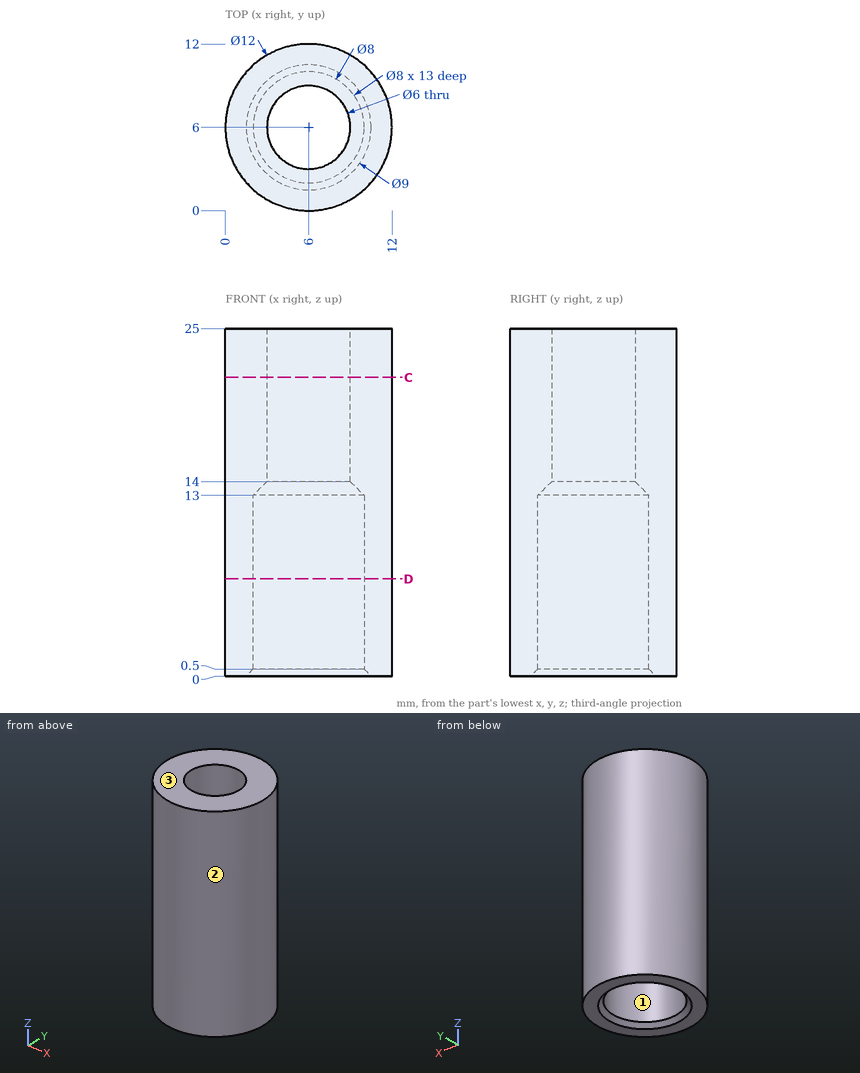
Here's the drawing with two shaded views (mm, measured from the low corner). I have some questions. Give positions to 0.01 mm unless a question says otherwise; leave off trailing zeros. Loops run counter-clockwise (first coordinate to the right, second up) from the corner with the lowest first, then second, coordinate; pieces in that order, holes last. Notation, with made-up numbers: M 53,31.5 L 95,31.5 A17 ccw 95,37.5 Z; hole C -18.75,-36.75 d6. An arc over 180 degrees is marked long. One line per item, written item: value.
(1) I need wall thicknesses on line 1 (Y direction, x = 6, z = 9.25); line 2 (Y direction, x = 5.5, z = 21.25); line 3 (X direction, y = 3.75, z = 6.75). Which ranges of each line are inside material? Lowest first, please.
Returned:
line 1: 0 to 2, 10 to 12
line 2: 0.02 to 3.04, 8.96 to 11.98
line 3: 0.44 to 2.69, 9.31 to 11.56
(2) We'd pull the mould along Y, two halves only. Please class the marked faces 1, 2 and 3: released by +Y, released by -Y, zero draft, split by the parting line, or undercut.
Returned:
face 1: undercut
face 2: split by the parting line
face 3: zero draft
(3) Suppose I cut it at C-C on z = 21.5. List the corners of the cut face in (x, y) for me.
Returned:
outline: C 6,6 d12; hole C 6,6 d6
(4) Will these pins go through, and if not, where does the flat tip stop? pin 1 (1 mm diameter, centred on y = 7, z = 20, fed in from +X); pin 2 (2.5 mm diameter, centred on x = 6, y = 4, fed in from -Z); pin 3 (1 mm diameter, centred on y = 10, z = 14.5, fed in from -X).
Returned:
pin 1: x = 11.98
pin 2: z = 13.75
pin 3: x = 1.13
(5) Suppose I cut it at D-D on z = 7. List the corners of the cut face in (x, y) for me.
Returned:
outline: C 6,6 d12; hole C 6,6 d8
